Check sheet for the drawn part. Datum: minimum x, y, z corner. Units: mm. A direction names the side the tool comes from. Give positions to 0.01 mm unless a question says otherwise; leave off trailing zeros. Loops run counter-clockwise (first coordinate to the right, second up) from the corner with the lowest first, then second, coordinate; pieces in that order, holes last.
1. Go/stop test with flat-tipped pins: pin 1 Ø3 at (x, z) = (76.5, 6) entering from -Y; pin 2 Ø4 at (y, z) = (44, 3.5) entering from +X; pin 3 Ø2 at (y, z) = (18.5, 3.5) entering from -X. Record where each tip stops, or that it passes through.
2. Cross-section at C-C, the plane y = 29. Record the cut outline in (x, z).
3. Tool access check on the marked faces 1 and 2. Record the directions out of +Z, -Z, +X, -X, +Y, -Y that give a thin tool (end or side, any length) a straight path to the whole face; none if there is none.
4. Cross-section at A-A, the plane x = 137.5. Record the cut outline in (y, z).
5. Cross-section at D-D, the plane x = 85. Record the cut outline in (y, z), plus the area to 3 significant figures.
6. Cross-section at B-B, the plane z = 4. Record the cut outline in (x, y).
7. Material ranges on L1, parallel to Y at x = 102, z = 6.5; L2, parallel to X at y = 40, z = 3; L3, parallel to X at y = 26.5, z = 2.5, recorded low to high.
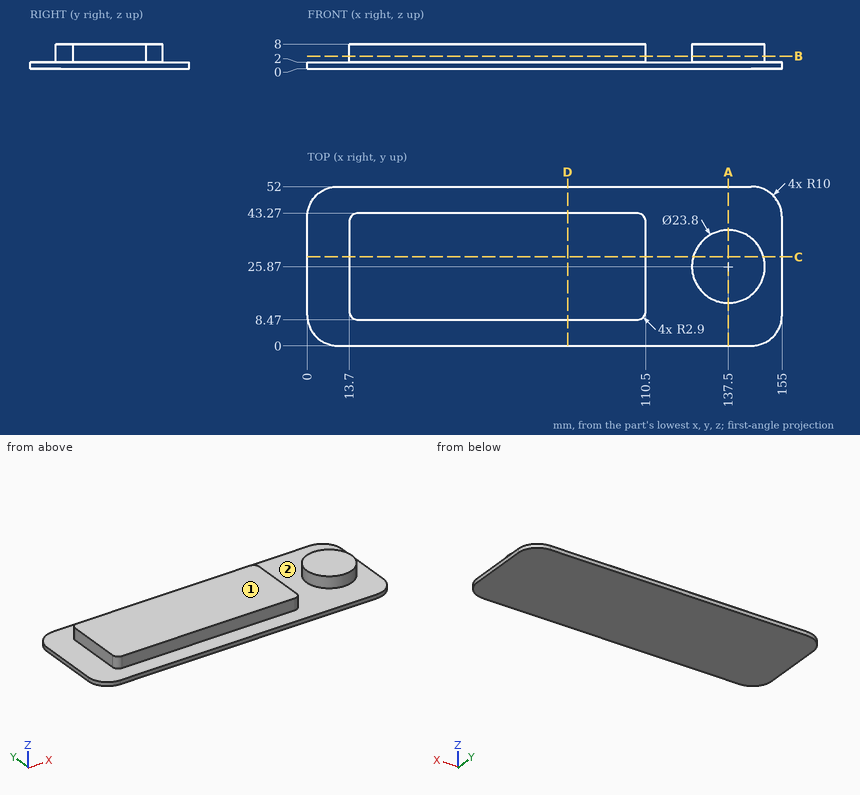
Result:
1. pin 1: stops at y = 8.47
1. pin 2: stops at x = 154.98
1. pin 3: stops at x = 13.7
2. outline: (0, 0) - (155, 0) - (155, 2) - (148.98, 2) - (148.98, 8) - (126.02, 8) - (126.02, 2) - (110.5, 2) - (110.5, 8) - (13.7, 8) - (13.7, 2) - (0, 2) - close
3. face 1: +Z, +X, -X, +Y, -Y
3. face 2: +Z
4. outline: (0, 0) - (52, 0) - (52, 2) - (37.77, 2) - (37.77, 8) - (13.97, 8) - (13.97, 2) - (0, 2) - close
5. outline: (0, 0) - (52, 0) - (52, 2) - (43.27, 2) - (43.27, 8) - (8.47, 8) - (8.47, 2) - (0, 2) - close
5. area: 313 mm2
6. outline: (13.7, 11.37) arc R2.9 ccw to (16.6, 8.47) - (107.6, 8.47) arc R2.9 ccw to (110.5, 11.37) - (110.5, 40.37) arc R2.9 ccw to (107.6, 43.27) - (16.6, 43.27) arc R2.9 ccw to (13.7, 40.37) - close; circle Ø23.8 at (137.5, 25.87)
7. L1: y = 8.47 to 43.27
7. L2: x = 13.7 to 110.5
7. L3: x = 13.7 to 110.5, 125.62 to 149.38
